from build123d import *

# Parameters (mm, degrees)
SKETCH_W        = 40
SKETCH_H        = 20
SKETCH_R        = 2
PAD_DEPTH       = 5
PAD001_DEPTH    = 40
FILLET_R        = 4
CHAMFER_SIZE    = 1
CHAMFER001_SIZE = 1.5


with BuildPart() as part:
    # Sketch → Pad (new body)
    with BuildSketch(Plane.XZ):
        Rectangle(SKETCH_W, SKETCH_H)
        with Locations((0, 5)):
            Circle(SKETCH_R, mode=Mode.SUBTRACT)
    extrude(amount=PAD_DEPTH)

    # Sketch001 (on Face7 of Pad) → Pad001 (join)
    with BuildSketch(Plane.XZ.offset(5)):
        with BuildLine():
            add(Edge.make_bspline(
                [(-20, -5.78744), (-20.688593, -0.934238), (0, 0)],
                knots=[0, 0, 0, 1, 1, 1], degree=2))
            add(Edge.make_bspline(
                [(20, -5.78744), (20.688593, -0.934238), (0, 0)],
                knots=[0, 0, 0, 1, 1, 1], degree=2))
            add(Edge.make_bspline(
                [(20, -5.78744), (19.908007, -9.418864), (0, -10)],
                knots=[0, 0, 0, 1, 1, 1], degree=2))
            add(Edge.make_bspline(
                [(-20, -5.78744), (-19.908007, -9.418864), (0, -10)],
                knots=[0, 0, 0, 1, 1, 1], degree=2))
        make_face()
    extrude(amount=PAD001_DEPTH)

    # Fillet
    fillet_edges = [part.edges().sort_by_distance(p)[0] for p in [
        (20, -2.5, 10),
        (20, -2.5, -10),
        (-20, -2.5, 10),
        (-20, -2.5, -10),
    ]]
    fillet(fillet_edges, radius=FILLET_R)

    # Chamfer
    chamfer_edges = [part.edges().sort_by_distance(p)[0] for p in [
        (10.984514, -45, -0.988644),
        (-10.984514, -45, -0.988644),
        (-10.562912, -45, -9.332673),
        (10.562912, -45, -9.332673),
    ]]
    chamfer(chamfer_edges, length=CHAMFER_SIZE)

    # Chamfer001
    chamfer001_edges = [part.edges().sort_by_distance(p)[0] for p in [
        (-2, -5, 5),
    ]]
    chamfer(chamfer001_edges, length=CHAMFER001_SIZE)


solid = part.part
Can you work these out from the model? Positions are in its coordinate system, mm. A direction names the side the tool comes from. Give positions to 0.01 mm unless a question says otherwise; leave off trailing zeros. Order: outer loops, then holes, each group sorted by start corner. A loop starts at its lowest first (then second) coordinate and runs counter-clockwise, first axis right, second up. Notation, with made-up numbers: (52, 2.5) - (66, 2.5) arc R21 ccw to (66, 7.5) - close; hole circle Ø10 at (-26, -34). An arc over 180 degrees is marked (long way). Write each question's results on one line, items separated by ' | '.
1) I'm going to push flat-ended pins straight in: pin 1 Ø2.5 at (y, z) = (-3.5, 0.5) entering from +X; pin 2 Ø1 at (x, y) = (1, -9) entering from +Z; pin 3 Ø10 at (x, y) = (-9.5, -9.5) entering from -Z; pin 4 Ø4.5 at (x, z) = (3, 2) entering from -Y. Where does each tip first touch, or does it pass through?
Final values:
pin 1: stops at x = 20 | pin 2: stops at z = -0.02 | pin 3: stops at z = -10 | pin 4: stops at y = -44.11
2) Suppose I cut it at A-A, the plane z = 5. Write out the boundary of the cut face in (x, y), then the cut area to 3 significant figures.
Final values:
outline: (-20, -5) - (-3.5, -5) - (-2, -3.5) - (-2, 0) - (-20, 0) - close; (2, -3.5) - (3.5, -5) - (20, -5) - (20, 0) - (2, 0) - close | area: 178 mm^2
3) Please list where these lines run through material, in increasing order: line 1 along Z through (x, y) = (0, -0.8); line 2 along Y through (x, z) = (11.5, 6); line 3 along Z through (x, y) = (18, -34). Write a range as [from, to].
Final values:
line 1: z = [-10, 3], [7, 10] | line 2: y = [-5, 0] | line 3: z = [-7.76, -2.94]
4) On a 3-axis mill with a long thin cutter (end or side, diameter ignored), from which of +Z, -Z, +X, -X, +Y, -Y can I reach the whole of each face in a straight line? I mean faces 5 (the face through (14, -5, -9)), 6 (the face through (0, 0, 0)). Say none if no direction works.
Final values:
face 5: -Z, +X, -Y | face 6: +Z, -Z, +X, -X, +Y
5) If we mould it in two halves opening along Z, with no side actions, what happens to faces 1 (the face through (0, -2, 7)), 2 (the face through (-14, -5, -9)), 3 (the face through (-18.859, -2.535, -8.797)), 4 (the face through (18.797, -2.535, 8.859))? For each: pulls with the +Z half, pulls with the -Z half, needs draft (parallel to the pull), parting line crosses it, or undercut.
Final values:
face 1: undercut | face 2: needs draft | face 3: pulls with the -Z half | face 4: pulls with the +Z half
